Design review of the part built by this model. Coordinates are the model's own, in mm. Coordinates: 2 decimals unless noted, no trailing zeros. Loops run counter-clockwise (first coordinate to the right, second up) from the corner with the lowest first, then second, coordinate; pieces in that order, holes last. Notation, with made-up numbers: M 40,32.25 L 70,32.25 A15 ccw 70,44.25 Z; hole C -23,64.25 d3. An arc over 180 degrees is marked long. Write item = value, one per line. Start each with the question number.
```python
from build123d import *

# Parameters (mm, degrees)
F1_DEPTH    = 25
F2_T1_DEPTH = 34.5185252635
F2_T3_DEPTH = 40
F2_T5_DEPTH = 25.7185484132


# Not quite as in the source:
# - a fillet or chamfer that OpenCascade refuses, or shapes differently, is made with other operations: its cross-section is extruded or revolved along the edge and cut away or added


with BuildPart() as f1:
    # F0 (on Front) → F1 (new body)
    with BuildSketch(Plane.XZ):
        with BuildLine():
            Line((-7, 0), (0, 0))
            Line((0, 0), (0, 380))
            Line((0, 380), (-7, 380))
            ThreePointArc((-7, 380), (-33.9910126529, 307.7803129177), (-48, 231.9651017804))
            Line((-48, 231.9651017804), (-48, 190))
            Line((-48, 190), (-48, 148.0348982196))
            ThreePointArc((-48, 148.0348982196), (-33.9910126529, 72.2196870823), (-7, 0))
        make_face()
    extrude(amount=F1_DEPTH)

    # F2: fillet of radius 3 on 5 edges, made by hand

    # F2_s2 → F2_t1 (cut)
    with BuildSketch(Plane.XZ.offset(-4.7592626318)):
        with BuildLine():
            ThreePointArc((-7.8159850821, 378.2800403279), (-6.7089962565, 379.533783829), (-5.1027772465, 380))
            Line((-5.1027772465, 380), (-7, 380))
            ThreePointArc((-7, 380), (-7.408920068, 379.1404602023), (-7.8159850821, 378.2800403279))
        make_face()
        with BuildLine():
            ThreePointArc((-7.8159850821, 1.7199596721), (-6.7089962565, 0.466216171), (-5.1027772465, 0))
            Line((-5.1027772465, 0), (-7, 0))
            ThreePointArc((-7, 0), (-7.408920068, 0.8595397977), (-7.8159850821, 1.7199596721))
        make_face()
    extrude(amount=F2_T1_DEPTH, mode=Mode.SUBTRACT)

    # F2_s4 → F2_t3 (cut)
    with BuildSketch(Plane.XZ.offset(-7.5)):
        with BuildLine():
            ThreePointArc((-3, 380), (-0.8786796564, 379.1213203436), (0, 377))
            Line((0, 377), (0, 380))
            Line((0, 380), (-3, 380))
        make_face()
        with BuildLine():
            ThreePointArc((0, 3), (-0.8786796564, 0.8786796564), (-3, 0))
            Line((-3, 0), (0, 0))
            Line((0, 0), (0, 3))
        make_face()
    extrude(amount=F2_T3_DEPTH, mode=Mode.SUBTRACT)

    # F2_s6 → F2_t5 (cut)
    with BuildSketch(Plane.XZ.offset(-0.3592742066)):
        with BuildLine():
            ThreePointArc((-47.9863097291, 232.1081578861), (-47.9965754777, 231.9651832447), (-48, 231.8218814431))
            Line((-48, 231.8218814431), (-48, 231.9651017804))
            ThreePointArc((-48, 231.9651017804), (-47.9931606883, 232.0366303906), (-47.9863097291, 232.1081578861))
        make_face()
    extrude(amount=F2_T5_DEPTH, mode=Mode.SUBTRACT)


solid = f1.part
```
(1) To check wall thickness, follow L1, parallel to X at y = -1.5, z = 21; L2, parallel to Z at x = -9.5, y = -11.75; L3, parallel to X at y = -19.25, z = 272.5. State the ranges of each line that lie inside material, in increasing order.
(2) Take a section at B-B (x = -13). State the section outline as (y, z) points.
(3) Take a section at A-A (y = -17.25). State the section outline as (x, z) points, plus the area to 3 significant figures.
(4) Take a section at C-C (z = 141). State the section outline as (x, y) points, plus the area to 3 significant figures.
(5) Insertion check: pin 1 (6 mm diameter, centred on x = -18, y = -2.5, fed in from -Z); pin 2 (5 mm diameter, centred on x = -20, y = -16.5, fed in from -Z); pin 3 (3 mm diameter, centred on x = -13, y = -16, fed in from -Z). Each pin has a flat end and moves straight along its axis. Give the tip position at first contact, or say it passes through.
Results list:
q1.L1 = -16.35 to 0
q1.L2 = 5.33 to 374.67
q1.L3 = -42.22 to 0
q2.outline = M -25,13.12 L 0,13.12 L 0,366.88 L -25,366.88 Z
q3.outline = M -48,148.03 A441.27 ccw -7.82,1.72 A3 ccw -5.1,0 L -3,0 A3 ccw 0,3 L 0,377 A3 ccw -3,380 L -5.1,380 A3 ccw -7.82,378.28 A441.27 ccw -47.99,232.11 A3 ccw -48,231.82 Z
q3.area = 13,500 mm^2
q4.outline = M -47.27,-25 L 0,-25 L 0,0 L -47.27,0 Z
q4.area = 1,180 mm^2
q5.pin_1 = 17.77
q5.pin_2 = 23.79
q5.pin_3 = 9.74
